from build123d import *

# Parameters (mm, degrees)
EXTRUDE_1_DEPTH          = 3
CUT_EXTRUDE_1_REACH      = 66.195
SKETCH_3_R               = 3.25
CUT_EXTRUDE_2_DEPTH      = 0.8
CUT_EXTRUDE_START        = -2.2
SKETCH_3_2_R             = 3.25
CUT_EXTRUDE_3_DEPTH      = 0.8
CUT_EXTRUDE_4_DEPTH      = 0.8
SKETCH_5_W               = 7
SKETCH_5_H               = 4
CUT_EXTRUDE_6_DEPTH      = 0.8
MIRROR_2_COPY_1_REACH    = 66.195
MIRROR_2_COPY_2_SKETCH_R = 3.25
MIRROR_2_COPY_2_DEPTH    = 0.8
MIRROR_START             = -2.2
MIRROR_2_COPY_3_SKETCH_R = 3.25
MIRROR_2_COPY_3_DEPTH    = 0.8


with BuildPart() as part:
    # 草图1 → 凸台-拉伸1 (new body)
    with BuildSketch(Plane.XY):
        with BuildLine():
            Line((0, 4), (60, 4))
            ThreePointArc((60, 4), (64, 0), (60, -4))
            Line((60, -4), (0, -4))
            ThreePointArc((0, -4), (-4, 0), (0, 4))
        make_face()
    extrude(amount=-EXTRUDE_1_DEPTH)

    # 草图2 → 切除-拉伸1 (cut, up to next)
    with BuildSketch(Plane.XY, mode=Mode.PRIVATE) as cut_extrude_1_sk1:
        with BuildLine():
            Line((1.322875656, -1.5), (2.883140649, -1.5))
            ThreePointArc((2.883140649, -1.5), (3.25, 0), (2.883140649, 1.5))
            Line((2.883140649, 1.5), (1.322875656, 1.5))
            ThreePointArc((1.322875656, 1.5), (0, 2), (-1.322875656, 1.5))
            Line((-1.322875656, 1.5), (-2.883140649, 1.5))
            ThreePointArc((-2.883140649, 1.5), (-3.25, 0), (-2.883140649, -1.5))
            Line((-2.883140649, -1.5), (-1.322875656, -1.5))
            ThreePointArc((-1.322875656, -1.5), (0, -2), (1.322875656, -1.5))
        make_face()
    cut_extrude_1_tool1 = extrude(cut_extrude_1_sk1.sketch, amount=-CUT_EXTRUDE_1_REACH, mode=Mode.PRIVATE) & part.part
    cut_extrude_1 = cut_extrude_1_tool1.solids().sort_by_distance((0, 0, 0))[0]
    add(cut_extrude_1, mode=Mode.SUBTRACT)

    # 草图3 → 切除-拉伸2 (cut)
    with BuildSketch(Plane.XY):
        Circle(SKETCH_3_R)
    cut_extrude_2 = extrude(amount=-CUT_EXTRUDE_2_DEPTH, mode=Mode.SUBTRACT)

    # 草图3<2> → 切除-拉伸3 (cut)
    with BuildSketch(Plane.XY.offset(CUT_EXTRUDE_START)):
        Circle(SKETCH_3_2_R)
    cut_extrude_3 = extrude(amount=-CUT_EXTRUDE_3_DEPTH, mode=Mode.SUBTRACT)

    # 草图4 → 切除-拉伸4 (cut)
    with BuildSketch(Plane.XY):
        with BuildLine():
            Line((3.464101615, 2), (11.535898385, 2))
            ThreePointArc((11.535898385, 2), (11, 0), (11.535898385, -2))
            Line((11.535898385, -2), (3.464101615, -2))
            ThreePointArc((3.464101615, -2), (4, 0), (3.464101615, 2))
        make_face()
    cut_extrude_4 = extrude(amount=-CUT_EXTRUDE_4_DEPTH, mode=Mode.SUBTRACT)

    # 草图5 → 切除-拉伸6 (cut)
    with BuildSketch(Plane(origin=(0, 0, -3), x_dir=(-1, 0, 0), z_dir=(0, 0, -1))):
        with Locations((-7.5, 0)):
            Rectangle(SKETCH_5_W, SKETCH_5_H)
    cut_extrude_6 = extrude(amount=-CUT_EXTRUDE_6_DEPTH, mode=Mode.SUBTRACT)

    # 镜向1: 切除-拉伸1, 切除-拉伸2, 切除-拉伸3 across plane
    add(cut_extrude_1.mirror(Plane(origin=(7.5, 0, 0), x_dir=(0, 0, 1), z_dir=(1, 0, 0))), mode=Mode.SUBTRACT)
    add(cut_extrude_2.mirror(Plane(origin=(7.5, 0, 0), x_dir=(0, 0, 1), z_dir=(1, 0, 0))), mode=Mode.SUBTRACT)
    add(cut_extrude_3.mirror(Plane(origin=(7.5, 0, 0), x_dir=(0, 0, 1), z_dir=(1, 0, 0))), mode=Mode.SUBTRACT)

    # 镜向2: 切除-拉伸1, 切除-拉伸2, 切除-拉伸3 across plane
    add(cut_extrude_1.mirror(Plane(origin=(22.5, 0, 0), x_dir=(0, 0, 1), z_dir=(1, 0, 0))), mode=Mode.SUBTRACT)
    add(cut_extrude_2.mirror(Plane(origin=(22.5, 0, 0), x_dir=(0, 0, 1), z_dir=(1, 0, 0))), mode=Mode.SUBTRACT)
    add(cut_extrude_3.mirror(Plane(origin=(22.5, 0, 0), x_dir=(0, 0, 1), z_dir=(1, 0, 0))), mode=Mode.SUBTRACT)

    # 镜向2 copy 1 sketch → 镜向2 copy 1 (cut, up to next)
    with BuildSketch(Plane(origin=(30, 0, 0), x_dir=(1, 0, 0), z_dir=(0, 0, 1)), mode=Mode.PRIVATE) as mirror_2_copy_1_sk1:
        with BuildLine():
            Line((1.322875656, -1.5), (2.883140649, -1.5))
            ThreePointArc((2.883140649, -1.5), (3.25, 0), (2.883140649, 1.5))
            Line((2.883140649, 1.5), (1.322875656, 1.5))
            ThreePointArc((1.322875656, 1.5), (0, 2), (-1.322875656, 1.5))
            Line((-1.322875656, 1.5), (-2.883140649, 1.5))
            ThreePointArc((-2.883140649, 1.5), (-3.25, 0), (-2.883140649, -1.5))
            Line((-2.883140649, -1.5), (-1.322875656, -1.5))
            ThreePointArc((-1.322875656, -1.5), (0, -2), (1.322875656, -1.5))
        make_face()
    mirror_2_copy_1_tool1 = extrude(mirror_2_copy_1_sk1.sketch, amount=-MIRROR_2_COPY_1_REACH, mode=Mode.PRIVATE) & part.part
    add(mirror_2_copy_1_tool1.solids().sort_by_distance((30, 0, 0))[0], mode=Mode.SUBTRACT)

    # 镜向2 copy 2 sketch → 镜向2 copy 2 (cut)
    with BuildSketch(Plane(origin=(30, 0, 0), x_dir=(1, 0, 0), z_dir=(0, 0, 1))):
        Circle(MIRROR_2_COPY_2_SKETCH_R)
    extrude(amount=-MIRROR_2_COPY_2_DEPTH, mode=Mode.SUBTRACT)

    # 镜向2 copy 3 sketch → 镜向2 copy 3 (cut)
    with BuildSketch(Plane(origin=(30, 0, 0), x_dir=(1, 0, 0), z_dir=(0, 0, 1)).offset(MIRROR_START)):
        Circle(MIRROR_2_COPY_3_SKETCH_R)
    extrude(amount=-MIRROR_2_COPY_3_DEPTH, mode=Mode.SUBTRACT)

    # 镜向3: 切除-拉伸4, 切除-拉伸6 across plane
    add(cut_extrude_4.mirror(Plane(origin=(15, 0, 0), x_dir=(0, 0, 1), z_dir=(1, 0, 0))), mode=Mode.SUBTRACT)
    add(cut_extrude_6.mirror(Plane(origin=(15, 0, 0), x_dir=(0, 0, 1), z_dir=(1, 0, 0))), mode=Mode.SUBTRACT)

    # 镜向4: 切除-拉伸4, 切除-拉伸6 across plane
    add(cut_extrude_4.mirror(Plane(origin=(22.5, 0, 0), x_dir=(0, 0, 1), z_dir=(1, 0, 0))), mode=Mode.SUBTRACT)
    add(cut_extrude_6.mirror(Plane(origin=(22.5, 0, 0), x_dir=(0, 0, 1), z_dir=(1, 0, 0))), mode=Mode.SUBTRACT)

    # 镜向5: 切除-拉伸1, 切除-拉伸2, 切除-拉伸3 across plane
    add(cut_extrude_1.mirror(Plane(origin=(30, 0, 0), x_dir=(0, 0, 1), z_dir=(1, 0, 0))), mode=Mode.SUBTRACT)
    add(cut_extrude_2.mirror(Plane(origin=(30, 0, 0), x_dir=(0, 0, 1), z_dir=(1, 0, 0))), mode=Mode.SUBTRACT)
    add(cut_extrude_3.mirror(Plane(origin=(30, 0, 0), x_dir=(0, 0, 1), z_dir=(1, 0, 0))), mode=Mode.SUBTRACT)

    # 镜向6: 切除-拉伸4, 切除-拉伸6 across plane
    add(cut_extrude_4.mirror(Plane(origin=(30, 0, 0), x_dir=(0, 0, 1), z_dir=(1, 0, 0))), mode=Mode.SUBTRACT)
    add(cut_extrude_6.mirror(Plane(origin=(30, 0, 0), x_dir=(0, 0, 1), z_dir=(1, 0, 0))), mode=Mode.SUBTRACT)


solid = part.part
Build history of the part. All positions in model axes, mm. A direction names the side the tool comes from. Round coordinates to 2 decimals unless told otherwise and drop trailing zeros. Write each loop counter-clockwise with the first axis right and the second up, starting at its lowest first coordinate (ties: lowest second). Pieces come first, ordered by that corner, then holes. Notation, with made-up numbers: (-7, -7.75) - (17, -7.75) arc R19 cw to (17, 5.25) - close; hole circle Ø3 at (20.25, 31.25). An arc over 180 degrees is marked (long way). Use CSV: the item, a comma, the result in double quotes.
(1) Pin check, flat tips, straight feed: P1, Ø0.5, axis at x = 1, y = 2.5, coming from the -Z side; P2, Ø0.9, axis at x = 16, y = -2, coming from the +Z side. Stop position of each tip, or through.
Response:
P1,"z = -2.2"
P2,"z = -0.8"
(2) Wall check: line 1 (X direction, y = 1.75, z = -0.95); line 2 (Y direction, x = 54, z = -2.3); line 3 (X direction, y = -1, z = -1.3). Give the ranges that are in metal, low to high.
Response:
line 1,"-3.6 to -0.97, 0.97 to 14.03, 15.97 to 29.03, 30.97 to 44.03, 45.97 to 59.03, 60.97 to 63.6"
line 2,"-4 to -2, 2 to 4"
line 3,"-3.87 to -3.09, 3.09 to 11.91, 18.09 to 26.91, 33.09 to 41.91, 48.09 to 56.91, 63.09 to 63.87"
(3) 3-axis set-ups, long thin cutter, end or side, ignore diameter. For faces 5 (the flat face through (0, -2.4, -2.2)), 6 (the flat face through (0, -2.4, -0.8)), 7 (the cylindrical face through (0, 2, -1)): which of +Z, -Z, +X, -X, +Y, -Y reach the whole face in a straight line?
Response:
face 5,"-Z"
face 6,"+Z"
face 7,"+Z, -Z"
(4) Band-saw the part on B-B (y = 0). Give the number of separate pieces and of enclosed holes in the cut face, plus the area to 3 significant figures.
Response:
separate pieces,"6"
enclosed holes,"0"
area,"61.7 mm²"
(5) Band-saw the part on A-A (x = 39). Write the cut outline in (y, z).
Response:
outline,"(-4, -3) - (-2, -3) - (-2, -2.2) - (2, -2.2) - (2, -3) - (4, -3) - (4, 0) - (2, 0) - (2, -0.8) - (-2, -0.8) - (-2, 0) - (-4, 0) - close"
(6) Mould opens along Y. For faces 1 (the flat face through (30, -2.4, -0.8)), 2 (the flat face through (33, 2, 0)), 3 (the flat face through (2, -1.5, -1)), 4 (the flat face through (30, 4, -1)) say: pulls with the +Y half, pulls with the -Y half, needs draft (parallel to the pull), parting line crosses it, or undercut.
Response:
face 1,"undercut"
face 2,"needs draft"
face 3,"undercut"
face 4,"pulls with the +Y half"
